Could you check a few things on this drawing? It's one solid part, dimensions in mm from its lowest x, y, z. Round coordinates to 2 decimals unless told otherwise and drop trailing zeros. Loops run counter-clockwise (first coordinate to the right, second up) from the corner with the lowest first, then second, coordinate; pieces in that order, holes last. Notation, with made-up numbers: (-3.75, 14) -> (27.25, 14) arc R14 cw to (27.25, 31) -> close; hole circle Ø2 at (16, -37). An arc over 180 degrees is marked (long way). Use one line per item in the form item = value. Start each with the question number.
Item 1: If we section it at A-A (x = 49): Write out the boundary of the cut face in (y, z), then the cut area to 3 significant figures.
Item 2: If I drill on L1, parallel to X at y = 89, z = 1.95; L2, parallel to X at y = 90.5, z = 1.85 (1 decimal); L3, parallel to Y at x = 53, z = 3.3, over which ranges is the centre line in solid material (lowest first)? Write a range as [from, to].
Item 3: If we section it at B-B (y = 65): Write out the boundary of the cut face in (x, z), then the cut area to 3 significant figures.
Item 4: If we section it at C-C (y = 123): Write out the boundary of the cut face in (x, z), then the cut area to 3 significant figures.
Item 5: I'm going to push flat-ended pins straight in: pin 1 Ø4 at (x, y) = (106.01, 106.01) entering from -Z; pin 2 Ø1 at (y, z) = (112.5, 3.5) entering from -X. Where does each tip first touch, or does it pass through?
Item 6: If we section it at D-D (z = 3.15): State how many separate pieces and enclosed holes the cut face has, then the cut area to 3 significant figures.
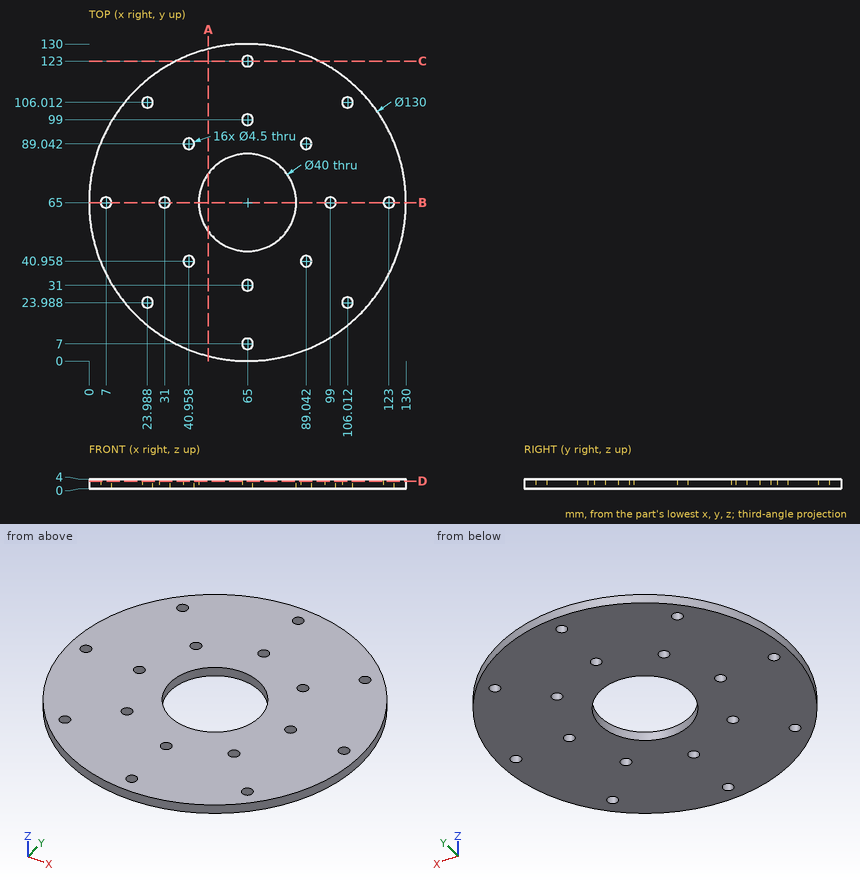
Values found:
q1.outline = (2, 0) -> (53, 0) -> (53, 4) -> (2, 4) -> close; (77, 0) -> (128, 0) -> (128, 4) -> (77, 4) -> close
q1.area = 408 mm2
q2.L1 = [4.59, 38.71], [43.21, 86.79], [91.29, 125.41]
q2.L2 = [5.2, 39.2], [42.7, 87.3], [90.8, 124.8]
q2.L3 = [1.12, 49], [81, 128.88]
q3.outline = (0, 0) -> (4.75, 0) -> (4.75, 4) -> (0, 4) -> close; (9.25, 0) -> (28.75, 0) -> (28.75, 4) -> (9.25, 4) -> close; (33.25, 0) -> (45, 0) -> (45, 4) -> (33.25, 4) -> close; (85, 0) -> (96.75, 0) -> (96.75, 4) -> (85, 4) -> close; (101.25, 0) -> (120.75, 0) -> (120.75, 4) -> (101.25, 4) -> close; (125.25, 0) -> (130, 0) -> (130, 4) -> (125.25, 4) -> close
q3.area = 288 mm2
q4.outline = (35.66, 0) -> (62.75, 0) -> (62.75, 4) -> (35.66, 4) -> close; (67.25, 0) -> (94.34, 0) -> (94.34, 4) -> (67.25, 4) -> close
q4.area = 217 mm2
q5.pin_1 = through
q5.pin_2 = 20.1
q6.separate_pieces = 1
q6.enclosed_holes = 17
q6.area = 11,800 mm2
